Geometry: final body of the model. Coordinates: model frame, mm. A direction names the side the tool comes from. Give positions to 0.01 mm unless a question says otherwise; leave off trailing zeros. Write each loop counter-clockwise with the first axis right and the second up, starting at its lowest first coordinate (ties: lowest second). Pieces come first, ordered by that corner, then holes. Notation, with made-up numbers: (69.25, 56) -> (103.25, 56) arc R24 cw to (103.25, 94) -> close; hole circle Ø6 at (82.5, 82.25). An arc over 180 degrees is marked (long way). Answer in a Markdown table with one row per item. Add a question column.
Item 1: Draft query along X for faces 6 (the flat face through (0, 32, -23)), 7 (the cylindrical face through (-28, 42, 21)), 8 (the cylindrical face through (-3.263, 45.356, -14.692)). Return one class per face: +X half, -X half, draft (parallel to the pull), parting line (faces both ways), or undercut.
Item 2: Section query A-A on z = 0. Output: boundary loops of the cut face in (x, y).
Item 3: Section query D-D on x = 7. Output: boundary loops of the cut face in (y, z).
Item 4: Access query for faces 1 (the flat face through (15, 0, 5)), 2 (the flat face through (25, 74.5, 0)), 3 (the cylindrical face through (-28.472, 72.034, -1.253)), 4 (the cylindrical face through (10.382, 15.776, -19.961)), 5 (the flat face through (-25, 85.7, 0)). Directions: +Z, -Z, +X, -X, +Y, -Y. A direction counts if a zero-diameter tool reaches every point of the face in a straight line with its end or side. Return the directions, or none.
Item 5: Section query B-B on x = 0. Output: boundary loops of the cut face in (y, z), plus the area to 3 significant figures.
Item 6: Material intervals for probe 1 along Z at (x, y) = (0, 30); probe 2 along Z at (x, y) = (0, 55); probe 3 along Y at (x, z) = (7, 32.5), sorted ascending. Write a range as from..to.
Item 7: Section query C-C on y = 23. Output: boundary loops of the cut face in (x, z), plus the area to 3 significant figures.
Item 8: First-contact query: P1, Ø6, axis at x = 18, y = 64.5, coming from the -Z side; P2, Ø3, axis at x = -7.5, y = 18.5, coming from the +Z side; P3, Ø12.5, axis at y = 78.5, z = 1.5, coming from the +X side; P4, Ø21, axis at x = -1.5, z = 14.5, coming from the +Y side. Flat tips, straight axial feed; report the tip coordinate or a pass-through.
```python
from build123d import *

# Parameters (mm, degrees)
SKETCH1_R            = 35
BOSS_EXTRUDE1_DEPTH  = 92
SKETCH2_OUTSIDE_W    = 99.028
SKETCH2_OUTSIDE_H    = 99.028
SKETCH2_OUTSIDE_R    = 28.5
CUT_EXTRUDE1_DEPTH   = 40.5
SKETCH3_OUTSIDE_W    = 99.028
SKETCH3_OUTSIDE_H    = 99.028
SKETCH3_OUTSIDE_R    = 22.5
CUT_EXTRUDE2_DEPTH   = 32
SKETCH4_R            = 15.05
CUT_EXTRUDE3_DEPTH   = 93
SKETCH5_W            = 5
SKETCH5_H            = 11.2
TESTINGFEATURE_DEPTH = 36


with BuildPart() as part:
    # Sketch1 → Boss-Extrude1 (new body)
    with BuildSketch(Plane(origin=(0, 0, 0), x_dir=(1, 0, 0), z_dir=(0, 1, 0))):
        Circle(SKETCH1_R)
    extrude(amount=BOSS_EXTRUDE1_DEPTH)

    # Sketch2 outside → Cut-Extrude1 (cut)
    with BuildSketch(Plane(origin=(0, 92, 0), x_dir=(1, 0, 0), z_dir=(0, 1, 0))):
        Rectangle(SKETCH2_OUTSIDE_W, SKETCH2_OUTSIDE_H)
        Circle(SKETCH2_OUTSIDE_R, mode=Mode.SUBTRACT)
    extrude(amount=-CUT_EXTRUDE1_DEPTH, mode=Mode.SUBTRACT)

    # Sketch3 outside → Cut-Extrude2 (cut)
    with BuildSketch(Plane.XZ):
        Rectangle(SKETCH3_OUTSIDE_W, SKETCH3_OUTSIDE_H)
        Circle(SKETCH3_OUTSIDE_R, mode=Mode.SUBTRACT)
    extrude(amount=-CUT_EXTRUDE2_DEPTH, mode=Mode.SUBTRACT)

    # Sketch4 → Cut-Extrude3 (cut, through all)
    with BuildSketch(Plane.XZ):
        Circle(SKETCH4_R)
    extrude(amount=-CUT_EXTRUDE3_DEPTH, mode=Mode.SUBTRACT)

    # Sketch5 → TestingFeature (cut, symmetric)
    with BuildSketch(Plane.XY):
        with Locations((26, 80.1)):
            Rectangle(SKETCH5_W, SKETCH5_H)
    testingfeature = extrude(amount=TESTINGFEATURE_DEPTH, both=True, mode=Mode.SUBTRACT)

    # Mirror1: TestingFeature across plane
    add(testingfeature.mirror(Plane(origin=(0, 0, 0), x_dir=(0, 0, 1), z_dir=(1, 0, 0))), mode=Mode.SUBTRACT)


solid = part.part
```
Findings below:
| question | item | result |
|---|---|---|
| 1 | face 6 | draft |
| 1 | face 7 | parting line |
| 1 | face 8 | undercut |
| 2 | outline | (-35, 32) -> (-22.5, 32) -> (-22.5, 0) -> (-15.05, 0) -> (-15.05, 92) -> (-28.5, 92) -> (-28.5, 85.7) -> (-23.5, 85.7) -> (-23.5, 74.5) -> (-28.5, 74.5) -> (-28.5, 51.5) -> (-35, 51.5) -> close; (15.05, 0) -> (22.5, 0) -> (22.5, 32) -> (35, 32) -> (35, 51.5) -> (28.5, 51.5) -> (28.5, 74.5) -> (23.5, 74.5) -> (23.5, 85.7) -> (28.5, 85.7) -> (28.5, 92) -> (15.05, 92) -> close |
| 3 | outline | (0, -21.38) -> (32, -21.38) -> (32, -34.29) -> (51.5, -34.29) -> (51.5, -27.63) -> (92, -27.63) -> (92, -13.32) -> (0, -13.32) -> close; (0, 13.32) -> (92, 13.32) -> (92, 27.63) -> (51.5, 27.63) -> (51.5, 34.29) -> (32, 34.29) -> (32, 21.38) -> (0, 21.38) -> close |
| 4 | face 1 | +Z, -Z, +X, -X, -Y |
| 4 | face 2 | +Z, -Z, +X |
| 4 | face 3 | +Y |
| 4 | face 4 | -Y |
| 4 | face 5 | +Z, -Z, -X |
| 5 | outline | (0, -22.5) -> (32, -22.5) -> (32, -35) -> (51.5, -35) -> (51.5, -28.5) -> (92, -28.5) -> (92, -15.05) -> (0, -15.05) -> close; (0, 15.05) -> (92, 15.05) -> (92, 28.5) -> (51.5, 28.5) -> (51.5, 35) -> (32, 35) -> (32, 22.5) -> (0, 22.5) -> close |
| 5 | area | 2,340 mm^2 |
| 6 | probe 1 | z = -22.5..-15.05, 15.05..22.5 |
| 6 | probe 2 | z = -28.5..-15.05, 15.05..28.5 |
| 6 | probe 3 | y = 32..51.5 |
| 7 | outline | circle Ø45 at (0, 0); hole circle Ø30.1 at (0, 0) |
| 7 | area | 879 mm^2 |
| 8 | P1 | stops at z = -24.23 |
| 8 | P2 | stops at z = 21.69 |
| 8 | P3 | stops at x = 28.5 |
| 8 | P4 | stops at y = 92 |
